Part model, mm, in its own coordinate system. A direction names the side the tool comes from. Round coordinates to 2 decimals unless told otherwise and drop trailing zeros. Loops run counter-clockwise (first coordinate to the right, second up) from the corner with the lowest first, then second, coordinate; pieces in that order, holes last. Notation, with made-up numbers: (80, 3.25) -> (87, 3.25) arc R4 cw to (87, 8.25) -> close; hole circle Ø7 at (60, 84). An arc over 180 degrees is marked (long way). Answer as CSV lines item,"result".
from build123d import *

# Parameters (mm, degrees)
SKETCH_1_W          = 12.25
SKETCH_1_H          = 11.3
EXTRUDE_1_DEPTH     = 2.15
SKETCH_2_W          = 1.5
SKETCH_2_H          = 11.3
EXTRUDE_2_DEPTH     = 3.85
SKETCH_5_W          = 9.25
SKETCH_5_H          = 11.5
CUT_EXTRUDE_1_DEPTH = 1
SKETCH_8_W          = 1.6
SKETCH_8_H          = 11.3
EXTRUDE_5_DEPTH     = 0.7
SKETCH_9_W          = 1.6
SKETCH_9_H          = 11.3
EXTRUDE_6_DEPTH     = 0.7
FILLET_8_R          = 0.3
SKETCH_11_W         = 12.25
SKETCH_11_H         = 4.85
CUT_EXTRUDE_2_DEPTH = 2
SKETCH_12_W         = 12.25
SKETCH_12_H         = 4.85
CUT_EXTRUDE_3_DEPTH = 2
SKETCH_13_W         = 1.15
SKETCH_13_H         = 11.3
EXTRUDE_7_DEPTH     = 0.5
SKETCH_14_W         = 1.15
SKETCH_14_H         = 11.3
EXTRUDE_8_DEPTH     = 0.5
FILLET_9_R          = 0.5
FILLET_10_R         = 0.7
FILLET_11_R         = 0.75


with BuildPart() as part:
    # 스케치1 → 보스-돌출1 (new body)
    with BuildSketch(Plane.XY):
        Rectangle(SKETCH_1_W, SKETCH_1_H)
    extrude(amount=EXTRUDE_1_DEPTH)

    # 스케치2 → 보스-돌출2 (add)
    with BuildSketch(Plane.XY.offset(2.15)):
        with Locations((-5.375, 0)):
            Rectangle(SKETCH_2_W, SKETCH_2_H)
        with Locations((5.375, 0)):
            Rectangle(SKETCH_2_W, SKETCH_2_H)
    extrude(amount=EXTRUDE_2_DEPTH)

    # 스케치5 → 컷-돌출1 (cut)
    with BuildSketch(Plane.XY.offset(2.15)):
        Rectangle(SKETCH_5_W, SKETCH_5_H)
    extrude(amount=-CUT_EXTRUDE_1_DEPTH, mode=Mode.SUBTRACT)

    # 스케치8 → 보스-돌출5 (add)
    with BuildSketch(Plane(origin=(-4.625, 0, 0), x_dir=(0, 0, -1), z_dir=(1, 0, 0))):
        with Locations((-5.2, 0)):
            Rectangle(SKETCH_8_W, SKETCH_8_H)
    extrude(amount=EXTRUDE_5_DEPTH)

    # 스케치9 → 보스-돌출6 (add)
    with BuildSketch(Plane.ZY.offset(-4.625)):
        with Locations((5.2, 0)):
            Rectangle(SKETCH_9_W, SKETCH_9_H)
    extrude(amount=EXTRUDE_6_DEPTH)

    # 필렛8
    fillet_8_edges = [part.edges().sort_by_distance(p)[0] for p in [
        (4.625, 0, 1.15),
        (-4.625, 0, 1.15),
    ]]
    fillet(fillet_8_edges, radius=FILLET_8_R)

    # 스케치11 → 컷-돌출2 (cut)
    with BuildSketch(Plane(origin=(0, 5.65, 0), x_dir=(1, 0, 0), z_dir=(0, 1, 0))):
        with Locations((0, -3.575)):
            Rectangle(SKETCH_11_W, SKETCH_11_H)
    extrude(amount=-CUT_EXTRUDE_2_DEPTH, mode=Mode.SUBTRACT)

    # 스케치12 → 컷-돌출3 (cut)
    with BuildSketch(Plane.XZ.offset(5.65)):
        with Locations((0, 3.575)):
            Rectangle(SKETCH_12_W, SKETCH_12_H)
    extrude(amount=-CUT_EXTRUDE_3_DEPTH, mode=Mode.SUBTRACT)

    # 스케치13 → 보스-돌출7 (add)
    with BuildSketch(Plane(origin=(6.125, 0, 0), x_dir=(0, 0, -1), z_dir=(1, 0, 0))):
        with Locations((-0.575, 0)):
            Rectangle(SKETCH_13_W, SKETCH_13_H)
    extrude(amount=EXTRUDE_7_DEPTH)

    # 스케치14 → 보스-돌출8 (add)
    with BuildSketch(Plane.ZY.offset(6.125)):
        with Locations((0.575, 0)):
            Rectangle(SKETCH_14_W, SKETCH_14_H)
    extrude(amount=EXTRUDE_8_DEPTH)

    # 필렛9
    fillet_9_edges = [part.edges().sort_by_distance(p)[0] for p in [
        (6.125, 0, 1.15),
        (-6.125, 0, 1.15),
    ]]
    fillet(fillet_9_edges, radius=FILLET_9_R - 0.0001)  # a hair under: the kernel refuses the full size

    # 필렛10
    fillet_10_edges = [part.edges().sort_by_distance(p)[0] for p in [
        (-3.925, 0, 6),
        (-3.925, 0, 4.4),
        (3.925, 0, 4.4),
        (3.925, 0, 6),
    ]]
    fillet(fillet_10_edges, radius=FILLET_10_R - 0.0001)  # a hair under: the kernel refuses the full size

    # 필렛11
    fillet_11_edges = [part.edges().sort_by_distance(p)[0] for p in [
        (6.625, -5.65, 0.575),
        (6.625, 5.65, 0.575),
        (-6.625, 5.65, 0.575),
        (-6.625, -5.65, 0.575),
    ]]
    fillet(fillet_11_edges, radius=FILLET_11_R)


solid = part.part
Q1. Drop flat-ended pins along their axis: P1, Ø1.3, axis at y = -1, z = 3, coming from the +X side (3 decimals); P2, Ø0.9, axis at y = -0.5, z = 2.5, coming from the -X side (3 decimals); P3, Ø1.5, axis at x = -1.5, z = 2, coming from the -Y side; P4, Ø3, axis at x = -5.5, z = 3.5, coming from the +Y side. Give the stop position or say it passes through.
Geometry results:
P1,"x = 6.125"
P2,"x = -6.125"
P3,"through"
P4,"y = 3.65"
Q2. Saw through at C-C, the plane x = 5.5. Write the cut outline in (y, z), then the cut area to 3 significant figures.
Geometry results:
outline,"(-5.65, 0) -> (5.65, 0) -> (5.65, 1.15) -> (3.65, 1.15) -> (3.65, 6) -> (-3.65, 6) -> (-3.65, 1.15) -> (-5.65, 1.15) -> close"
area,"48.4 mm2"
Q3. Two-plate mould, pull along Z, no slides. Class faces 1 (the face through (-4.625, 0, 3)), 2 (the face through (5, 0, 6)), 3 (the face through (4.625, 0, 3)), 4 (the face through (5, 3.65, 4)): pulls with the +Z half, pulls with the -Z half, needs draft (parallel to the pull), parting line crosses it, or undercut.
Geometry results:
face 1,"undercut"
face 2,"pulls with the +Z half"
face 3,"undercut"
face 4,"needs draft"
Q4. Which spindle directions (+Z, -Z, +X, -X, +Y, -Y) get a long thin tool onto all of the face, cutting with end or side? Do faces 5 (the face through (6.125, 0, 4)), 6 (the face through (-6.125, 0, 4)), 7 (the face through (-5, -3.65, 4)). Say none if no direction does.
Geometry results:
face 5,"+Z, +X, +Y, -Y"
face 6,"+Z, -X, +Y, -Y"
face 7,"+Z, +X, -X, -Y"
Q5. Saw through at B-B, the plane z = 3.9. Write the cut outline in (x, y) (3 decimals), then the cut area to 3 significant figures.
Geometry results:
outline,"(-6.125, -3.65) -> (-4.625, -3.65) -> (-4.625, 3.65) -> (-6.125, 3.65) -> close; (4.625, -3.65) -> (6.125, -3.65) -> (6.125, 3.65) -> (4.625, 3.65) -> close"
area,"21.9 mm2"
Q6. Drill centre lines: line 1 along X through (y, z) = (1.5, 3.25) (3 decimals); line 2 along Z through (x, y) = (3, -1.75); line 3 along Y through (x, z) = (5.5, 4.55). Where is each one in solid material? Low to high.
Geometry results:
line 1,"-6.125 to -4.625, 4.625 to 6.125"
line 2,"0 to 1.15"
line 3,"-3.65 to 3.65"
